Source: CAD feature listing. Evaluate the final solid. Frame: model axes, mm. A direction names the side the tool comes from. Give positions to 0.01 mm unless a question says otherwise; leave off trailing zeros. Order: outer loops, then holes, each group sorted by start corner. A loop starts at its lowest first (then second) coordinate and runs counter-clockwise, first axis right, second up.
from build123d import *

# Parameters (mm, degrees)
BOSS_EXTRUDE1_DEPTH      = 10
BOSS_EXTRUDE1_DEPTH_BACK = 10
CUT_EXTRUDE1_DEPTH       = 213.726165923
CUT_EXTRUDE1_DEPTH_BACK  = 213.726165923
SKETCH2_W                = 18
SKETCH2_H                = 18


with BuildPart() as part:
    # Sketch1 → Boss-Extrude1 (new, two sides: drawn at the far end of the back side and taken through both)
    with BuildSketch(Plane.XY.offset(-BOSS_EXTRUDE1_DEPTH_BACK)):
        with BuildLine():
            Line((-7.098078142, 152.098078142), (-116.934338078, 21.200320767))
            Line((-116.934338078, 21.200320767), (-101.613449216, 8.344568573))
            Line((-101.613449216, 8.344568573), (-96.5092206, 14.427551362))
            ThreePointArc((-96.5092206, 14.427551362), (-48.790839046, 3.626817852), (0, 0))
            Line((0, 0), (3.5, 0))
            Line((3.5, 0), (3.5, 141.5))
            Line((3.5, 141.5), (-7.098078142, 152.098078142))
        make_face()
        with BuildLine():
            Line((-3.5, 7), (-3.5, 125.271624157))
            Line((-3.5, 125.271624157), (-91.625019277, 20.248315836))
            ThreePointArc((-91.625019277, 20.248315836), (-48.02157631, 10.570542672), (-3.5, 7))
        make_face(mode=Mode.SUBTRACT)
    extrude(amount=BOSS_EXTRUDE1_DEPTH + BOSS_EXTRUDE1_DEPTH_BACK)

    # Sketch2 → Cut-Extrude1 (cut, two sides: drawn at the far end of the back side and taken through both)
    with BuildSketch(Plane(origin=(-37.875331553, -45.138062449, 0), x_dir=(-0.7660444431189823, 0.6427876096865343, 0), z_dir=(-0.6427876096865343, -0.7660444431189825, 0)).offset(-CUT_EXTRUDE1_DEPTH_BACK)):
        with Locations((93.204203405, 0)):
            Rectangle(SKETCH2_W, SKETCH2_H)
    extrude(amount=CUT_EXTRUDE1_DEPTH + CUT_EXTRUDE1_DEPTH_BACK, mode=Mode.SUBTRACT)


solid = part.part
1) Ray query, L1, parallel to X at y = 44.5, z = 4; L2, parallel to Z at x = -26, y = 127; L3, parallel to Y at x = -10, z = 2.25. Return the intervals inside material, ascending.
Checks:
L1: x = -97.38 to -96.08, -72.58 to -71.28, -3.5 to 3.5
L2: z = -10 to -9, 9 to 10
L3: y = 0.15 to 7.14, 117.53 to 119.08, 147.08 to 148.64
2) Section query A-A on z = -1.75. Output: boundary loops of the cut face in (x, y), and give its area (3 significant figures).
Checks:
outline: (-116.93, 21.2) - (-116.17, 20.56) - (-6.39, 151.39) - (-7.1, 152.1) - close; (-102.38, 8.99) - (-101.61, 8.34) - (-96.51, 14.43) arc R330 ccw to (0, 0) - (3.5, 0) - (3.5, 135.17) - close; hole (-91.63, 20.25) arc R323.02 ccw to (-3.5, 7) - (-3.5, 125.27) - close
area: 1,880 mm2
3) Section query C-C on y = 52. Output: boundary loops of the cut face in (x, z).
Checks:
outline: (-91.09, -10) - (-64.98, -10) - (-64.98, 10) - (-91.09, 10) - close; (-3.5, -10) - (3.5, -10) - (3.5, 10) - (-3.5, 10) - close; hole (-89.78, -9) - (-66.29, -9) - (-66.29, 9) - (-89.78, 9) - close
4) Pull-direction query (Y, two-part tool) for faces 4 (the face through (-54, 81, -9)), 5 (the face through (3.5, 70, 0)), 6 (the face through (-48.7, 72.96, 0.13)), 7 (the face through (-99.1, 11.34, -0.14)); classes: +Y half, -Y half, draft (parallel to the pull), parting line (faces both ways), or undercut.
Checks:
face 4: undercut
face 5: draft
face 6: undercut
face 7: -Y half
5) Reachability of faces 1 (the face through (-48.64, 10.664, -0.14)), 2 (the face through (-49.47, 3.73, -0.14)), 3 (the face through (-60.5, 86.9, 0.1)) from +Z, -Z, +X, -X, +Y, -Y: full face, straight path, thin tool, end or side. Return the list, or none.
Checks:
face 1: +Z, -Z
face 2: +Z, -Z, -Y
face 3: none
6) Section query D-D on y = 12.5. Output: boundary loops of the cut face in (x, z), and give its area (3 significant figures).
Checks:
outline: (-106.57, -10) - (-98.13, -10) - (-98.13, 10) - (-106.57, 10) - (-106.57, 9) - (-99.43, 9) - (-99.43, -9) - (-106.57, -9) - close; (-89.97, -10) - (-59.46, -10) - (-59.46, 10) - (-89.97, 10) - close; (-3.5, -10) - (3.5, -10) - (3.5, 10) - (-3.5, 10) - close
area: 791 mm2
7) First-contact query: pin 1 Ø1.5 at (x, z) = (-72, 5) entering from +Y; pin 2 Ø4 at (y, z) = (78.5, -4.5) entering from -X; pin 3 Ø3 at (x, z) = (-18, 1) entering from +Y. Flat tips, straight axial feed; report the tip coordinate or a pass-through.
Checks:
pin 1: stops at y = 75.64
pin 2: stops at x = -70.53
pin 3: stops at y = 140.89
8) Section query B-B on x = -51.5. Output: boundary loops of the cut face in (y, z), and give its area (3 significant figures).
Checks:
outline: (4.04, -10) - (11.11, -10) - (11.11, 10) - (4.04, 10) - close; (68.07, -10) - (99.18, -10) - (99.18, 10) - (68.07, 10) - close; hole (69.62, -9) - (97.63, -9) - (97.63, 9) - (69.62, 9) - close
area: 260 mm2
